Build history of the part. All positions in model axes, mm. A direction names the side the tool comes from. Coordinates: 2 decimals unless noted, no trailing zeros. Write each loop counter-clockwise with the first axis right and the second up, starting at its lowest first coordinate (ties: lowest second). Pieces come first, ordered by that corner, then holes.
from build123d import *

# Parameters (mm, degrees)
SKETCH1_R           = 3.15
BOSS_EXTRUDE1_DEPTH = 5.9
CUT_EXTRUDE2_DEPTH  = 2.5


with BuildPart() as part:
    # Sketch1 → Boss-Extrude1 (new body)
    with BuildSketch(Plane.XY):
        with BuildLine():
            Line((23.375, -8), (-23.375, -8))
            ThreePointArc((-23.375, -8), (-31.375, 0), (-23.375, 8))
            Line((-23.375, 8), (23.375, 8))
            ThreePointArc((23.375, 8), (31.375, 0), (23.375, -8))
        make_face()
        with Locations((23.375, 0)):
            Circle(SKETCH1_R, mode=Mode.SUBTRACT)
        with Locations((-23.375, 0)):
            Circle(SKETCH1_R, mode=Mode.SUBTRACT)
    extrude(amount=BOSS_EXTRUDE1_DEPTH)

    # Sketch2 → Cut-Extrude2 (cut)
    with BuildSketch(Plane.XY):
        Polygon((23.375, 5.831237719), (18.325, 2.915618859), (18.325, -2.915618859), (23.375, -5.831237719), (28.425, -2.915618859), (28.425, 2.915618859), align=None)
    extrude(amount=CUT_EXTRUDE2_DEPTH, mode=Mode.SUBTRACT)


solid = part.part
(1) Slice it at D-D, the plane y = 5. List the corners of the cut face in (x, z).
(2) Slice it at B-B, the plane z = 4.6. List the corners of the cut face in (x, y) (3 decimals), and give its area (3 significant figures).
(3) Slice it at A-A, the plane y = 1.25. List the corners of the cut face in (x, z) (3 decimals), and give its area (3 significant figures).
(4) Slice it at C-C, the plane x = 21.5. List the corners of the cut face in (y, z).
(5) Probe L1, parallel to X at y = -2, z = 0.5 (3 decimals); L2, parallel to X at y = -2.75, z = 2 (3 decimals); L3, parallel to Y at x = -21, z = 0.75. List the from-to ranges inside material, lowest first.
(6) Two-plate mould, pull along Y, no slides. Class faces 1 (the cylindrical face through (-26.52, 0.14, 2.91)), 2 (the flat face through (0, -8, 3)), 3 (the flat face through (0, 0, 0)): pulls with the +Y half, pulls with the -Y half, needs draft (parallel to the pull), parting line crosses it, or undercut.
(7) 3-axis set-ups, long thin cutter, end or side, ignore diameter. For faces 4 (the cylindrical face through (-31.373, -0.176, 2.909)), 5 (the flat face through (21, -3, 2.5)): which of +Z, -Z, +X, -X, +Y, -Y reach the whole face in a straight line?
Results:
1. outline: (-29.62, 0) - (21.94, 0) - (21.94, 2.5) - (24.81, 2.5) - (24.81, 0) - (29.62, 0) - (29.62, 5.9) - (-29.62, 5.9) - close
2. outline: (-23.375, -8) - (23.375, -8) arc R8 ccw to (23.375, 8) - (-23.375, 8) arc R8 ccw to start; hole circle Ø6.3 at (-23.375, 0); hole circle Ø6.3 at (23.375, 0)
2. area: 887 mm2
3. outline: (-31.277, 0) - (-26.266, 0) - (-26.266, 5.9) - (-31.277, 5.9) - close; (-20.484, 0) - (18.325, 0) - (18.325, 2.5) - (20.484, 2.5) - (20.484, 5.9) - (-20.484, 5.9) - close; (26.266, 2.5) - (28.425, 2.5) - (28.425, 0) - (31.277, 0) - (31.277, 5.9) - (26.266, 5.9) - close
3. area: 290 mm2
4. outline: (-8, 0) - (-4.75, 0) - (-4.75, 2.5) - (-2.53, 2.5) - (-2.53, 5.9) - (-8, 5.9) - close; (2.53, 2.5) - (4.75, 2.5) - (4.75, 0) - (8, 0) - (8, 5.9) - (2.53, 5.9) - close
5. L1: x = -31.121 to -25.809, -20.941 to 18.325, 28.425 to 31.121
5. L2: x = -30.887 to -24.911, -21.839 to 18.325, 28.425 to 30.887
5. L3: y = -8 to -2.07, 2.07 to 8
6. face 1: undercut
6. face 2: pulls with the -Y half
6. face 3: needs draft
7. face 4: +Z, -Z, -X
7. face 5: -Z
